```python
from build123d import *

# Parameters (mm, degrees)
SKETCH1_W           = 25.4
SKETCH1_H           = 47.625
BOSS_EXTRUDE1_DEPTH = 3.175
SKETCH2_W           = 12.7
SKETCH2_H           = 3.175
CUT_EXTRUDE1_DEPTH  = 55.068301712
FILLET1_R           = 2.54


with BuildPart() as part:
    # Sketch1 → Boss-Extrude1 (new body)
    with BuildSketch(Plane(origin=(0, 0, 0), x_dir=(1, 0, 0), z_dir=(0, 1, 0))):
        with Locations((12.7, 23.8125)):
            Rectangle(SKETCH1_W, SKETCH1_H)
    extrude(amount=BOSS_EXTRUDE1_DEPTH)

    # Sketch2 → Cut-Extrude1 (cut, through all)
    with BuildSketch(Plane(origin=(0, 3.175, 0), x_dir=(1, 0, 0), z_dir=(0, 1, 0))):
        with Locations((12.7, 39.6875)):
            Rectangle(SKETCH2_W, SKETCH2_H)
    extrude(amount=-CUT_EXTRUDE1_DEPTH, mode=Mode.SUBTRACT)

    # Fillet1
    fillet1_edges = [part.edges().sort_by_distance(p)[0] for p in [
        (0, 1.5875, -47.625),
        (25.4, 1.5875, -47.625),
        (25.4, 1.5875, 0),
        (0, 1.5875, 0),
    ]]
    fillet(fillet1_edges, radius=FILLET1_R)


solid = part.part
```
Input: part model. Units: mm. Frame: model coordinates. A direction names the side the tool comes from. Coordinates: 2 decimals unless noted, no trailing zeros. Write each loop counter-clockwise with the first axis right and the second up, starting at its lowest first coordinate (ties: lowest second). Pieces come first, ordered by that corner, then holes. Notation, with made-up numbers: (12, 51) - (70, 51) arc R26 cw to (70, 69) - close; hole circle Ø10 at (86.5, 10.25). An arc over 180 degrees is marked (long way). Put each result on its own line as item: value. Start each with the question number.
1) Cut plane A-A (x = 8.25). Return the cut outline in (y, z) (3 decimals).
2) Ray query, L1, parallel to Z at x = 18.5, y = 0.45 (3 decimals); L2, parallel to X at y = 2, z = -38.5; L3, parallel to Z at x = 1.25, y = 1.05. Return the intervals inside material, ascending.
3) Contact query for a flat-ended pin moving along its axis: pin 1 (2 mm diameter, centred on x = 5, z = -15.5, fed in from -Y). Output: stop coordinate, or through.
4) Cut plane B-B (y = 0.9). Return the cut outline in (x, z) (3 decimals), plus the area to 3 significant figures.
5) Reachability of faces 1 (the face through (13, 2, -38.1)), 2 (the face through (0, 2, -24)) from +Z, -Z, +X, -X, +Y, -Y: full face, straight path, thin tool, end or side. Return the list, or none.
6) Mould query, pull axis Z, two halves, no side actions, for faces 3 (the face through (6.35, 2, -40)), 4 (the face through (13, 0, -24)), 5 (the face through (13, 2, -41.275)), 6 (the face through (13, 2, -47.625)). Classes: pulls with the +Z half, pulls with the -Z half, needs draft (parallel to the pull), parting line crosses it, or undercut.
Resolved:
1. outline: (0, -47.625) - (3.175, -47.625) - (3.175, -41.275) - (0, -41.275) - close; (0, -38.1) - (3.175, -38.1) - (3.175, 0) - (0, 0) - close
2. L1: z = -47.625 to -41.275, -38.1 to 0
2. L2: x = 0 to 6.35, 19.05 to 25.4
2. L3: z = -47.27 to -0.35
3. pin 1: stops at y = 0
4. outline: (0, -45.085) arc R2.54 ccw to (2.54, -47.625) - (22.86, -47.625) arc R2.54 ccw to (25.4, -45.085) - (25.4, -2.54) arc R2.54 ccw to (22.86, 0) - (2.54, 0) arc R2.54 ccw to (0, -2.54) - close; hole (6.35, -41.275) - (19.05, -41.275) - (19.05, -38.1) - (6.35, -38.1) - close
4. area: 1,160 mm2
5. face 1: +Y, -Y
5. face 2: +Z, -Z, -X, +Y, -Y
6. face 3: undercut
6. face 4: needs draft
6. face 5: undercut
6. face 6: pulls with the -Z half
